Source: CAD feature listing. Evaluate the final solid. Frame: model axes, mm. Face numbers are marked on the shaded views. A direction names the side the tool comes from. Give positions to 0.01 mm unless a question says otherwise; leave off trailing zeros. Loops run counter-clockwise (first coordinate to the right, second up) from the corner with the lowest first, then second, coordinate; pieces in that order, holes last. Notation, with made-up numbers: (49.25, 20) - (67.25, 20) arc R25 ccw to (67.25, 49) - close; hole circle Ø2 at (21.25, 80). An arc over 180 degrees is marked (long way). Put each result on its own line as item: value.
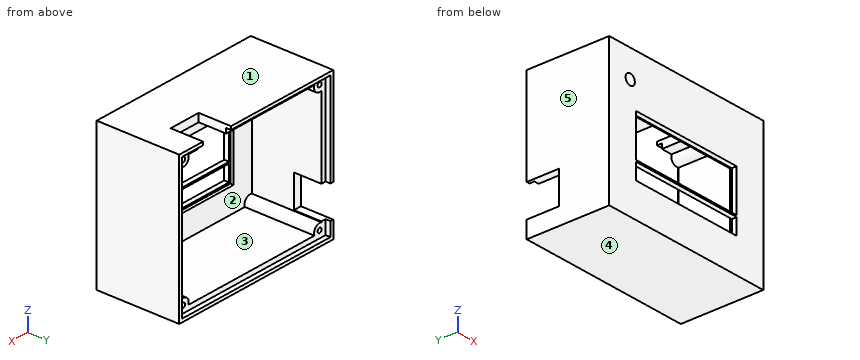
```python
from build123d import *

# Parameters (mm, degrees)
SKETCH1_W                  = 110
SKETCH1_H                  = 90
BOSS_EXTRUDE1_DEPTH        = 51
SKETCH2_W                  = 100
SKETCH2_H                  = 80
CUT_EXTRUDE1_DEPTH         = 46
SKETCH3_W                  = 106
SKETCH3_H                  = 3
CUT_EXTRUDE2_DEPTH         = 3
SKETCH5_W                  = 3
SKETCH5_H                  = 83
CUT_EXTRUDE3_DEPTH         = 3
SKETCH6_W                  = 103
SKETCH6_H                  = 3
CUT_EXTRUDE4_DEPTH         = 3
SKETCH7_W                  = 3
SKETCH7_H                  = 80
CUT_EXTRUDE5_DEPTH         = 3
SKETCH9_R                  = 4
BOSS_EXTRUDE2_DEPTH        = 43
SKETCH10_R                 = 4
BOSS_EXTRUDE3_DEPTH        = 43
M2_5_CLEARANCE_HOLE1_D     = 2.9
M2_5_CLEARANCE_HOLE1_DEPTH = 5
M2_5_CLEARANCE_HOLE1_TIP   = 0.871247898
SKETCH14_W                 = 20
SKETCH14_H                 = 20
CUT_EXTRUDE6_DEPTH         = 5
SKETCH15_W                 = 20
SKETCH15_H                 = 20
CUT_EXTRUDE7_DEPTH         = 5
SKETCH16_W                 = 72
SKETCH16_H                 = 26
CUT_EXTRUDE8_DEPTH         = 5
SKETCH17_W                 = 72
SKETCH17_H                 = 10
CUT_EXTRUDE9_DEPTH         = 5
M6_CLEARANCE_HOLE2_D       = 6.6
SKETCH22_W                 = 74
SKETCH22_H                 = 39
CUT_EXTRUDE10_DEPTH        = 2


with BuildPart() as part:
    # Sketch1 → Boss-Extrude1 (new body)
    with BuildSketch(Plane(origin=(0, 0, 0), x_dir=(1, 0, 0), z_dir=(0, 1, 0))):
        Rectangle(SKETCH1_W, SKETCH1_H)
    extrude(amount=BOSS_EXTRUDE1_DEPTH)

    # Sketch2 → Cut-Extrude1 (cut)
    with BuildSketch(Plane(origin=(0, 51, 0), x_dir=(1, 0, 0), z_dir=(0, 1, 0))):
        Rectangle(SKETCH2_W, SKETCH2_H)
    extrude(amount=-CUT_EXTRUDE1_DEPTH, mode=Mode.SUBTRACT)

    # Sketch3 → Cut-Extrude2 (cut)
    with BuildSketch(Plane(origin=(0, 51, 0), x_dir=(1, 0, 0), z_dir=(0, 1, 0))):
        with Locations((0, 41.5)):
            Rectangle(SKETCH3_W, SKETCH3_H)
    extrude(amount=-CUT_EXTRUDE2_DEPTH, mode=Mode.SUBTRACT)

    # Sketch5 → Cut-Extrude3 (cut)
    with BuildSketch(Plane(origin=(0, 51, 0), x_dir=(1, 0, 0), z_dir=(0, 1, 0))):
        with Locations((51.5, -1.5)):
            Rectangle(SKETCH5_W, SKETCH5_H)
    extrude(amount=-CUT_EXTRUDE3_DEPTH, mode=Mode.SUBTRACT)

    # Sketch6 → Cut-Extrude4 (cut)
    with BuildSketch(Plane(origin=(0, 51, 0), x_dir=(1, 0, 0), z_dir=(0, 1, 0))):
        with Locations((-1.5, -41.5)):
            Rectangle(SKETCH6_W, SKETCH6_H)
    extrude(amount=-CUT_EXTRUDE4_DEPTH, mode=Mode.SUBTRACT)

    # Sketch7 → Cut-Extrude5 (cut)
    with BuildSketch(Plane(origin=(0, 51, 0), x_dir=(1, 0, 0), z_dir=(0, 1, 0))):
        with Locations((-51.5, 0)):
            Rectangle(SKETCH7_W, SKETCH7_H)
    extrude(amount=-CUT_EXTRUDE5_DEPTH, mode=Mode.SUBTRACT)

    # Sketch9 → Boss-Extrude2 (add)
    with BuildSketch(Plane(origin=(0, 5, 0), x_dir=(1, 0, 0), z_dir=(0, 1, 0))):
        with Locations((-48.75, 38.75)):
            Circle(SKETCH9_R)
    extrude(amount=BOSS_EXTRUDE2_DEPTH)

    # Sketch10 → Boss-Extrude3 (add)
    with BuildSketch(Plane(origin=(0, 5, 0), x_dir=(1, 0, 0), z_dir=(0, 1, 0))):
        with Locations((48.75, 38.75)):
            Circle(SKETCH10_R)
        with Locations((48.75, -38.75)):
            Circle(SKETCH10_R)
        with Locations((-48.75, -38.75)):
            Circle(SKETCH10_R)
    extrude(amount=BOSS_EXTRUDE3_DEPTH)

    # M2.5 Clearance Hole1
    with Locations(Plane(origin=(0, 48, 0), x_dir=(1, 0, 0), z_dir=(0, 1, 0))):
        with Locations((-48.75, 38.75), (48.75, 38.75), (48.75, -38.75), (-48.75, -38.75)):
            Hole(M2_5_CLEARANCE_HOLE1_D / 2, depth=M2_5_CLEARANCE_HOLE1_DEPTH)
            with Locations((0, 0, -(M2_5_CLEARANCE_HOLE1_DEPTH + M2_5_CLEARANCE_HOLE1_TIP / 2))):  # 118° drill point
                Cone(0, M2_5_CLEARANCE_HOLE1_D / 2, M2_5_CLEARANCE_HOLE1_TIP, mode=Mode.SUBTRACT)

    # Sketch14 → Cut-Extrude6 (cut)
    with BuildSketch(Plane.ZY.offset(55)):
        with Locations((-24.5, 41)):
            Rectangle(SKETCH14_W, SKETCH14_H)
    extrude(amount=-CUT_EXTRUDE6_DEPTH, mode=Mode.SUBTRACT)

    # Sketch15 → Cut-Extrude7 (cut)
    with BuildSketch(Plane.XY.offset(45)):
        with Locations((28, 41)):
            Rectangle(SKETCH15_W, SKETCH15_H)
    extrude(amount=-CUT_EXTRUDE7_DEPTH, mode=Mode.SUBTRACT)

    # Sketch16 → Cut-Extrude8 (cut)
    with BuildSketch(Plane(origin=(0, 5, 0), x_dir=(1, 0, 0), z_dir=(0, 1, 0))):
        Rectangle(SKETCH16_W, SKETCH16_H)
    extrude(amount=-CUT_EXTRUDE8_DEPTH, mode=Mode.SUBTRACT)

    # Sketch17 → Cut-Extrude9 (cut)
    with BuildSketch(Plane.XZ):
        with Locations((0, -19)):
            Rectangle(SKETCH17_W, SKETCH17_H)
    extrude(amount=-CUT_EXTRUDE9_DEPTH, mode=Mode.SUBTRACT)

    # M6 Clearance Hole2 (through all)
    with Locations(Plane(origin=(0, 0, 0), x_dir=(-1, 0, 0), z_dir=(0, -1, 0))):
        with Locations((40, -28)):
            Hole(M6_CLEARANCE_HOLE2_D / 2)

    # Sketch22 → Cut-Extrude10 (cut)
    with BuildSketch(Plane(origin=(0, 5, 0), x_dir=(1, 0, 0), z_dir=(0, 1, 0))):
        with Locations((0, 5.5)):
            Rectangle(SKETCH22_W, SKETCH22_H)
    extrude(amount=-CUT_EXTRUDE10_DEPTH, mode=Mode.SUBTRACT)


solid = part.part
```
1) Section query A-A, the plane z = -2.5. Output: boundary loops of the cut face in (x, y), plus the area to 3 significant figures.
Check result:
outline: (-55, 0) - (-36, 0) - (-36, 3) - (-37, 3) - (-37, 5) - (-50, 5) - (-50, 48) - (-53, 48) - (-53, 51) - (-55, 51) - close; (36, 0) - (55, 0) - (55, 51) - (53, 51) - (53, 48) - (50, 48) - (50, 5) - (37, 5) - (37, 3) - (36, 3) - close
area: 628 mm²
2) Mould query, pull axis X, two halves, no side actions, for the marked faces 3, 4 and 5. Classes: pulls with the +X half, pulls with the -X half, needs draft (parallel to the pull), parting line crosses it, or undercut.
Check result:
face 3: undercut
face 4: needs draft
face 5: pulls with the -X half
3) Section query C-C, the plane y = 39. Output: boundary loops of the cut face in (x, z).
Check result:
outline: (-55, -45) - (55, -45) - (55, 45) - (38, 45) - (38, 40) - (44.95, 40) arc R4 ccw to (50, 34.95) - (50, -34.95) arc R4 ccw to (44.95, -40) - (-44.95, -40) arc R4 ccw to (-50, -34.95) - (-50, -34.5) - (-55, -34.5) - close; (-55, -14.5) - (-50, -14.5) - (-50, 34.95) arc R4 ccw to (-44.95, 40) - (18, 40) - (18, 45) - (-55, 45) - close
4) Section query D-D, the plane x = -41.5. Output: boundary loops of the cut face in (y, z).
Check result:
outline: (0, -45) - (51, -45) - (51, -43) - (48, -43) - (48, -40) - (5, -40) - (5, 25.06) - (0, 25.06) - close; (0, 30.94) - (5, 30.94) - (5, 40) - (48, 40) - (48, 43) - (51, 43) - (51, 45) - (0, 45) - close
5) Pin query (flat end, axial travel): P1, Ø3.5, axis at x = 48.75, z = -38.75, coming from the +Y side; P2, Ø2, axis at x = 0, z = 24.5, coming from the +Y side; P3, Ø3, axis at x = -34.5, z = -13, coming from the +Y side; P4, Ø4, axis at x = -40, z = 28, coming from the +Y side. Return the tip coordinate at first contact, or that it passes through.
Check result:
P1: y = 48
P2: y = 5
P3: y = 3
P4: through
6) Section query B-B, the plane x = -17. Output: boundary loops of the cut face in (y, z), plus the area to 3 significant figures.
Check result:
outline: (0, -45) - (51, -45) - (51, -43) - (48, -43) - (48, -40) - (5, -40) - (5, -25) - (3, -25) - (3, -24) - (0, -24) - close; (0, -14) - (3, -14) - (3, -13) - (0, -13) - close; (0, 13) - (3, 13) - (3, 14) - (5, 14) - (5, 40) - (48, 40) - (48, 43) - (51, 43) - (51, 45) - (0, 45) - close
area: 706 mm²
7) Access query for the marked faces 1 and 2. Directions: +Z, -Z, +X, -X, +Y, -Y. A direction counts if a zero-diameter tool reaches every point of the face in a straight line with its end or side. Return the directions, or none.
Check result:
face 1: +Z, +X, -X, +Y, -Y
face 2: +Y
8) Material intervals for line 1 along X through (y, z) = (45.75, -38.75); line 2 along X through (y, z) = (26.5, -25.5); line 3 along Z through (x, y) = (-13, 16.5), sorted ascending. Write a range as [from, to].
Check result:
line 1: [-55, -50.2], [-47.3, -44.75], [44.75, 47.3], [50.2, 55]
line 2: [-55, -50], [50, 55]
line 3: [-45, -40], [40, 45]
